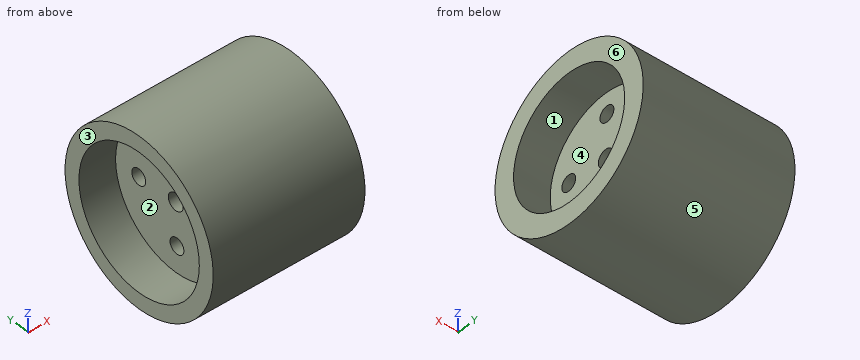
```python
from build123d import *

# Parameters (mm, degrees)
SKETCH4_R               = 1.5
CUT_EXTRUDE1_DEPTH      = 17
SKETCH5_R               = 12
SKETCH5_R_2             = 1.5
SKETCH5_R_3             = 1.6
BOSS_EXTRUDE1_DEPTH     = 2
CUT_EXTRUDE2_DEPTH      = 31.066592757
CUT_EXTRUDE2_DEPTH_BACK = 31.066592757
SKETCH6_W               = 2
SKETCH6_H               = 36


with BuildPart() as part:
    # Sketch3 → Revolve1 (revolve)
    with BuildSketch(Plane.XY, mode=Mode.PRIVATE) as revolve1_sk:
        Polygon((-7, 1.6), (6, 1.6), (6, 12), (15, 12), (15, 16), (-14, 16), (-14, 18), (-16, 18), (-16, 13), (-7, 13), align=None)
    revolve(revolve1_sk.sketch.rotate(Axis((0, 0, 0), (1, 0, 0)), 90), axis=Axis((0, 0, 0), (1, 0, 0)))

    # Sketch4 → Cut-Extrude1 (cut)
    with BuildSketch(Plane.ZY.offset(7)):
        with Locations((0.262567942, -7.995689969)):
            Circle(SKETCH4_R)
        with Locations((-7.995689969, -0.262567942)):
            Circle(SKETCH4_R)
        with Locations((-0.262567942, 7.995689969)):
            Circle(SKETCH4_R)
        with Locations((7.995689969, 0.262567942)):
            Circle(SKETCH4_R)
    extrude(amount=-CUT_EXTRUDE1_DEPTH, mode=Mode.SUBTRACT)

    # Sketch5 → Boss-Extrude1 (add)
    with BuildSketch(Plane(origin=(6, 0, 0), x_dir=(0, 0, -1), z_dir=(1, 0, 0))):
        with Locations(Location((0, 0, 0), (0, 0, 180))):
            Circle(SKETCH5_R)
        with Locations(Location((7.995689969, -0.262567942, 0), (0, 0, 180))):
            Circle(SKETCH5_R_2, mode=Mode.SUBTRACT)
        with Locations(Location((-0.262567942, -7.995689969, 0), (0, 0, 180))):
            Circle(SKETCH5_R_2, mode=Mode.SUBTRACT)
        with Locations(Location((-7.995689969, 0.262567942, 0), (0, 0, 180))):
            Circle(SKETCH5_R_2, mode=Mode.SUBTRACT)
        with Locations(Location((0.262567942, 7.995689969, 0), (0, 0, 180))):
            Circle(SKETCH5_R_2, mode=Mode.SUBTRACT)
        with Locations(Location((0, 0, 0), (0, 0, 180))):
            Circle(SKETCH5_R_3, mode=Mode.SUBTRACT)
    extrude(amount=BOSS_EXTRUDE1_DEPTH)

    # Sketch6 → Cut-Extrude2 (cut, two sides: drawn at the far end of the back side and taken through both)
    with BuildSketch(Plane.XY.offset(-CUT_EXTRUDE2_DEPTH_BACK)):
        with Locations((-15, 0)):
            Rectangle(SKETCH6_W, SKETCH6_H)
    extrude(amount=CUT_EXTRUDE2_DEPTH + CUT_EXTRUDE2_DEPTH_BACK, mode=Mode.SUBTRACT)


solid = part.part
```
Verification items for the finished model (mm, model axes). Face numbers are marked on the shaded views. A direction names the side the tool comes from. Give positions to 0.01 mm unless a question says otherwise; leave off trailing zeros. Order: outer loops, then holes, each group sorted by start corner. A loop starts at its lowest first (then second) coordinate and runs counter-clockwise, first axis right, second up. Notation, with made-up numbers: M 83.25,0.25 L 136.25,0.25 A28 cw 136.25,37.25 Z; hole C -23.5,-2.75 d7. An arc over 180 degrees is marked long. Return JSON: item names as keys, results as strings. Group by question number.
1) Section check B-B on y = 10.5. Record the cut outline in (x, z), and give its area (3 significant figures).
2) Section check C-C on x = -9.25. Record the cut outline in (y, z), and give its area (3 significant figures).
3) Access from +Z, -Z, +X, -X, +Y, -Y to the whole of each face (thin tool, end or side, straight path). Record for the marked faces 1, 2 and 3.
4) Section check A-A on z = -8.5. Record the cut outline in (x, y), and give its area (3 significant figures).
5) Mould release check, pull along Y, two halves, no side actions. Record for the marked faces 4, 5 and 6: pulls with the +Y half, pulls with the -Y half, needs draft (parallel to the pull), parting line crosses it, or undercut.
6) Section check D-D on z = 9. Record the cut outline in (x, y).
7) Go/stop test with flat-tipped pins: pin 1 Ø2 at (x, y) = (8, -4.5) entering from +Z; pin 2 Ø2 at (x, y) = (-10.5, -12) entering from -Z; pin 3 Ø8 at (x, y) = (1.5, 8) entering from -Z. Record where each tip stops, or that it passes through.
8) Scan lines: line 1 (Y direction, x = -10.5, z = 0); line 2 (X direction, y = -8, z = -10); line 3 (X direction, y = 3.5, z = -0.5). Record each from-to range of solid material in increasing order.
Answer block:
{
 "1": {"outline": "M -14,-12.07 L 15,-12.07 L 15,-5.81 L 8,-5.81 L 8,5.81 L 15,5.81 L 15,12.07 L -14,12.07 L -14,7.66 L -7,7.66 L -7,-7.66 L -14,-7.66 Z", "area": "512 mm^2"},
 "2": {"outline": "C 0,0 d32; hole C 0,0 d26", "area": "273 mm^2"},
 "3": {"face 1": "+X", "face 2": "-X", "face 3": "+Z, -Z, -X, +Y, -Y"},
 "4": {"outline": "M -14,-13.56 L 15,-13.56 L 15,-8.47 L 8,-8.47 L 8,-1.68 L -7,-1.68 L -7,-9.84 L -14,-9.84 Z; M -14,9.84 L -7,9.84 L -7,1.15 L 8,1.15 L 8,8.47 L 15,8.47 L 15,13.56 L -14,13.56 Z", "area": "488 mm^2"},
 "5": {"face 4": "undercut", "face 5": "parting line crosses it", "face 6": "needs draft"},
 "6": {"outline": "M -14,-13.23 L 15,-13.23 L 15,-7.94 L 8,-7.94 L 8,-0.85 L -7,-0.85 L -7,-9.38 L -14,-9.38 Z; M -14,9.38 L -7,9.38 L -7,1.38 L 8,1.38 L 8,7.94 L 15,7.94 L 15,13.23 L -14,13.23 Z"},
 "7": {"pin 1": "stops at z = 15.61", "pin 2": "stops at z = -11.62", "pin 3": "stops at z = -15.49"},
 "8": {"line 1": "y = -16 to -13, 13 to 16", "line 2": "x = -7 to 15", "line 3": "x = -7 to 8"}
}
